```python
from build123d import *

# Parameters (mm, degrees)
BOX_W             = 200
BOX_H             = 22
BOX_DEPTH         = 2.5
CYLINDER_R        = 2.25
CYLINDER_DEPTH    = 2.5
CYLINDER001_R     = 2.25
CYLINDER001_DEPTH = 2.5
CYLINDER003_R     = 1.3
CYLINDER003_DEPTH = 6
CYLINDER004_R     = 0.5
CYLINDER004_DEPTH = 2.5
BOX003_W          = 8
BOX003_H          = 22
BOX003_DEPTH      = 10
BOX004_W          = 101
BOX004_H          = 10
BOX004_DEPTH      = 2.5
BOX005_W          = 142
BOX005_H          = 7
BOX005_DEPTH      = 2.5
BOX006_W          = 8
BOX006_H          = 6
BOX006_DEPTH      = 10
BOX007_W          = 14
BOX007_H          = 4
BOX007_DEPTH      = 2.5


with BuildPart() as part:
    # Box → Box (join)
    with BuildSketch(Plane.XY):
        with Locations((100, 11)):
            Rectangle(BOX_W, BOX_H)
    extrude(amount=BOX_DEPTH)

    # Cylinder → Cylinder (cut)
    with BuildSketch(Plane(origin=(19.25, 16, 0), x_dir=(1, 0, 0), z_dir=(0, 0, 1))):
        Circle(CYLINDER_R)
    extrude(amount=CYLINDER_DEPTH, mode=Mode.SUBTRACT)

    # Cylinder001 → Cylinder001 (cut)
    with BuildSketch(Plane(origin=(188.25, 17, 0), x_dir=(1, 0, 0), z_dir=(0, 0, 1))):
        Circle(CYLINDER001_R)
    extrude(amount=CYLINDER001_DEPTH, mode=Mode.SUBTRACT)

    # Cylinder003 → Cylinder003 (join)
    with BuildSketch(Plane(origin=(145, 4.5, -5), x_dir=(1, 0, 0), z_dir=(0, 0, 1))):
        Circle(CYLINDER003_R)
    extrude(amount=CYLINDER003_DEPTH)

    # Cylinder004 → Cylinder004 (cut)
    with BuildSketch(Plane(origin=(30.25, 4.5, 2.5), x_dir=(1, 0, 0), z_dir=(0, 0, -1))):
        Circle(CYLINDER004_R)
    extrude(amount=CYLINDER004_DEPTH, mode=Mode.SUBTRACT)

    # Box003 → Box003 (cut)
    with BuildSketch(Plane(origin=(0.25, 22, 2.25), x_dir=(1, 0, 0), z_dir=(0, 0, -1))):
        with Locations((4, 11)):
            Rectangle(BOX003_W, BOX003_H)
    extrude(amount=BOX003_DEPTH, mode=Mode.SUBTRACT)

    # Box004 → Box004 (cut)
    with BuildSketch(Plane(origin=(37.25, 15, 2.5), x_dir=(1, 0, 0), z_dir=(0, 0, -1))):
        with Locations((50.5, 5)):
            Rectangle(BOX004_W, BOX004_H)
    extrude(amount=BOX004_DEPTH, mode=Mode.SUBTRACT)

    # Box005 → Box005 (cut)
    with BuildSketch(Plane(origin=(29.25, 22, 2.5), x_dir=(1, 0, 0), z_dir=(0, 0, -1))):
        with Locations((71, 3.5)):
            Rectangle(BOX005_W, BOX005_H)
    extrude(amount=BOX005_DEPTH, mode=Mode.SUBTRACT)

    # Box006 → Box006 (cut)
    with BuildSketch(Plane(origin=(29.25, 15, 2.5), x_dir=(1, 0, 0), z_dir=(0, 0, -1))):
        with Locations((4, 3)):
            Rectangle(BOX006_W, BOX006_H)
    extrude(amount=BOX006_DEPTH, mode=Mode.SUBTRACT)

    # Box007 → Box007 (cut)
    with BuildSketch(Plane(origin=(138.25, 15, 2.5), x_dir=(1, 0, 0), z_dir=(0, 0, -1))):
        with Locations((7, 2)):
            Rectangle(BOX007_W, BOX007_H)
    extrude(amount=BOX007_DEPTH, mode=Mode.SUBTRACT)


solid = part.part
```
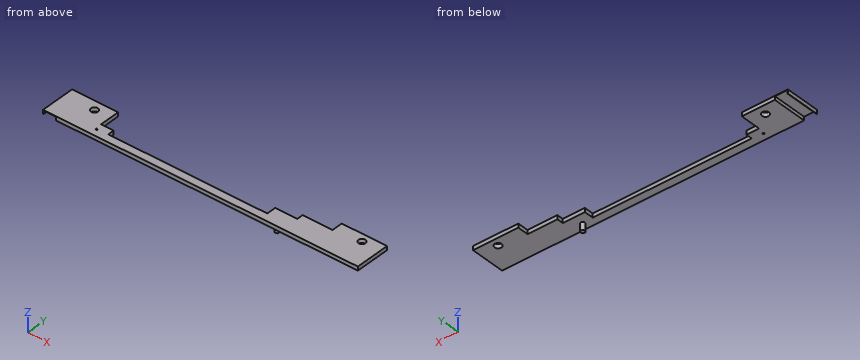
Can you work these out from the model? Positions are in its coordinate system, mm. Round coordinates to 2 decimals unless told otherwise and drop trailing zeros. Loops run counter-clockwise (first coordinate to the right, second up) from the corner with the lowest first, then second, coordinate; pieces in that order, holes last.
Item 1: Suppose I cut it at C-C, the plane x = 168. Write out the boundary of the cut face in (y, z), then the cut area to 3 significant figures.
Item 2: Please list where these lines run through material, in increasing order: L1, parallel to X at y = 4.5, z = 0.6; L2, parallel to Y at x = 19.25, z = 1; L3, parallel to Y at x = 30.25, z = 1.9.
Item 3: Suppose I cut it at B-B, the plane x = 71.5. Write out the boundary of the cut face in (y, z), then the cut area to 3 significant figures.
Item 4: Suppose I cut it at A-A, the plane x = 188.25. Write out the boundary of the cut face in (y, z).
Item 5: Will these pins go through, and if not, where does the flat tip stop? pin 1 Ø2 at (x, z) = (32, 1) entering from +Y; pin 2 Ø6 at (x, y) = (188.25, 17) entering from -Z; pin 3 Ø3 at (x, z) = (147.5, 1.5) entering from +Y.
Reported:
1. outline: (0, 0) - (15, 0) - (15, 2.5) - (0, 2.5) - close
1. area: 37.5 mm2
2. L1: x = 0 to 0.25, 8.25 to 29.75, 30.75 to 200
2. L2: y = 0 to 13.75, 18.25 to 22
2. L3: y = 0 to 4, 5 to 9
3. outline: (0, 0) - (5, 0) - (5, 2.5) - (0, 2.5) - close
3. area: 12.5 mm2
4. outline: (0, 0) - (14.75, 0) - (14.75, 2.5) - (0, 2.5) - close; (19.25, 0) - (22, 0) - (22, 2.5) - (19.25, 2.5) - close
5. pin 1: stops at y = 9
5. pin 2: stops at z = 0
5. pin 3: stops at y = 11
